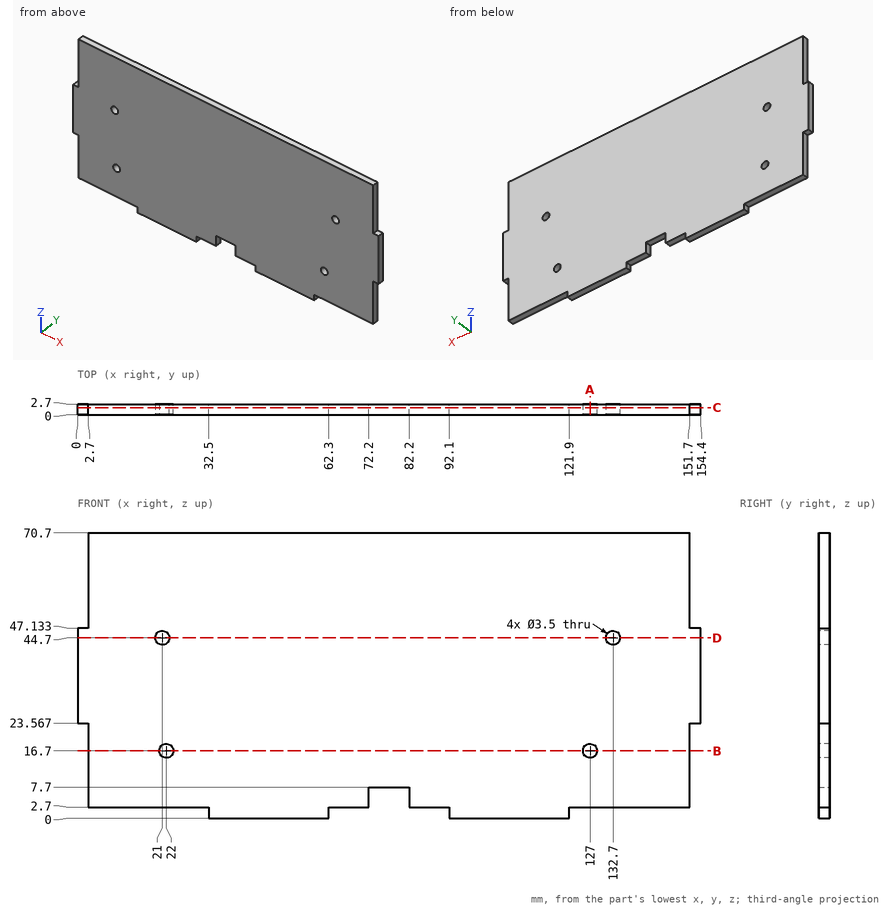
Input: dimensioned drawing with shaded views. Units: mm. Origin: part minimum x, y, z. Coordinates: 2 decimals unless noted, no trailing zeros. Write each loop counter-clockwise with the first axis right and the second up, starting at its lowest first coordinate (ties: lowest second). Pieces come first, ordered by that corner, then holes. Notation, with made-up numbers: M 66.5,17 L 82.5,17 A27 cw 82.5,33 Z; hole C 19,16.25 d10. An arc over 180 degrees is marked long. Use a Markdown table: item, result.
1) Section A-A, the plane x = 127. Output: boundary loops of the cut face in (y, z), then the cut area to 3 significant figures.
Conclusion:
| item | result |
|---|---|
| outline | M 0,2.7 L 2.7,2.7 L 2.7,14.95 L 0,14.95 Z; M 0,18.45 L 2.7,18.45 L 2.7,70.7 L 0,70.7 Z |
| area | 174 mm^2 |
2) Ray query, L1, parallel to X at y = 1.8, z = 44.7; L2, parallel to X at y = 2.2, z = 5.5; L3, parallel to Z at x = 127, y = 1.95. Return the intervals inside material, ascending.
Conclusion:
| item | result |
|---|---|
| L1 | x = 0 to 19.25, 22.75 to 130.95, 134.45 to 154.4 |
| L2 | x = 2.7 to 72.2, 82.2 to 151.7 |
| L3 | z = 2.7 to 14.95, 18.45 to 70.7 |
3) First-contact query: pin 1 Ø0.8 at (x, y) = (1, 1) entering from -Z; pin 2 Ø0.8 at (y, z) = (1, 58.5) entering from -X; pin 3 Ø2 at (x, z) = (132.7, 44.7) entering from +Y; pin 4 Ø0.8 at (x, y) = (66.5, 1) entering from -Z. Flat tips, straight axial feed; report the tip coordinate or a pass-through.
Conclusion:
| item | result |
|---|---|
| pin 1 | stops at z = 23.57 |
| pin 2 | stops at x = 2.7 |
| pin 3 | passes through |
| pin 4 | stops at z = 2.7 |
4) Section B-B, the plane z = 16.7. Output: boundary loops of the cut face in (x, y).
Conclusion:
| item | result |
|---|---|
| outline | M 2.7,0 L 20.25,0 L 20.25,2.7 L 2.7,2.7 Z; M 23.75,0 L 125.25,0 L 125.25,2.7 L 23.75,2.7 Z; M 128.75,0 L 151.7,0 L 151.7,2.7 L 128.75,2.7 Z |
5) Section D-D, the plane z = 44.7. Output: boundary loops of the cut face in (x, y), then the cut area to 3 significant figures.
Conclusion:
| item | result |
|---|---|
| outline | M 0,0 L 19.25,0 L 19.25,2.7 L 0,2.7 Z; M 22.75,0 L 130.95,0 L 130.95,2.7 L 22.75,2.7 Z; M 134.45,0 L 154.4,0 L 154.4,2.7 L 134.45,2.7 Z |
| area | 398 mm^2 |
6) Section C-C, the plane y = 1.8. Output: boundary loops of the cut face in (x, z), then the cut area to 3 significant figures.
Conclusion:
| item | result |
|---|---|
| outline | M 0,23.57 L 2.7,23.57 L 2.7,2.7 L 32.5,2.7 L 32.5,0 L 62.3,0 L 62.3,2.7 L 72.2,2.7 L 72.2,7.7 L 82.2,7.7 L 82.2,2.7 L 92.1,2.7 L 92.1,0 L 121.9,0 L 121.9,2.7 L 151.7,2.7 L 151.7,23.57 L 154.4,23.57 L 154.4,47.13 L 151.7,47.13 L 151.7,70.7 L 2.7,70.7 L 2.7,47.13 L 0,47.13 Z; hole C 21,44.7 d3.5; hole C 22,16.7 d3.5; hole C 127,16.7 d3.5; hole C 132.7,44.7 d3.5 |
| area | 10,300 mm^2 |
